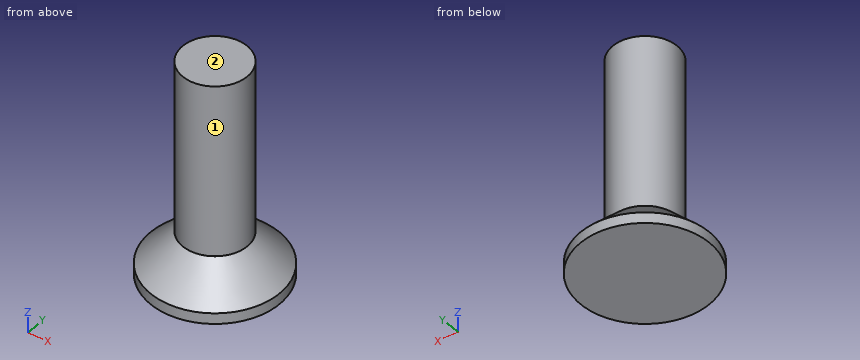
Autodesk Inventor part; units mm, degrees
ref_plane "YZ Plane" through (0, 0, 0) normal (1, 0, 0) x (0, 1, 0)
ref_plane "XZ Plane" through (0, 0, 0) normal (0, 1, 0) x (-1, 0, 0)
ref_plane "XY Plane" through (0, 0, 0) normal (0, 0, 1) x (1, 0, 0)
sketch "スケッチ1" plane through (0, 0, 0) normal (0, 0, 1) x (1, 0, 0)
  circle A0 centre (0, 0) radius 1.5
  dimension "d0" = 3
extrude "押し出し1" add sketch "スケッチ1" along normal blind 10
sketch "スケッチ2" plane through (0, 0, 0) normal (0, 0, -1) x (-1, 0, 0)
  circle A0 centre (0, 0) radius 3
  dimension "d3" = 6
extrude "押し出し2" add sketch "スケッチ2" against normal blind 2
thread "ねじ1"
chamfer "面取り1" distance 1.5 angle 45 1 edges at (3, 0, 2)
properties part number "ネジ皿m3,10" material "鋼、高強度、低合金"
Work out the finished part from the listing and answer in its coordinate system (mm). Face numbers are marked on the shaded views. A direction names the side the tool comes from. Give positions to 0.01 mm unless a question says otherwise; leave off trailing zeros. Order: outer loops, then holes, each group sorted by start corner. A loop starts at its lowest first (then second) coordinate and runs counter-clockwise, first axis right, second up. Notation, with made-up numbers: (41, 9.5) - (61, 9.5) arc R23 cw to (61, 24.5) - close; hole circle Ø6 at (13.25, 33.5). An arc over 180 degrees is marked (long way). Answer as CSV lines item,"result". Start each with the question number.
Q1. Given pin 1 Ø2 at (y, z) = (1.5, 3) entering from +X; pin 2 Ø1 at (x, z) = (0.5, 3) entering from -Y; pin 3 Ø1.5 at (x, y) = (2, -2) entering from +Z; pin 4 Ø3 at (x, y) = (0, -1.5) entering from -Z, each flat-ended and moving along its own axis, determine where each tip first touches the part or whether it passes through.
Q2. Find the intervals of material crossed by L1, parallel to Z at x = -2.15, y = -0.8; L2, parallel to Z at x = -0.85, y = -2.65; L3, parallel to Y at x = -1.15, z = 2.5, in increasing order. Write a range as [from, to].
Q3. For the marked faces 1 and 2, determine the directions among +Z, -Z, +X, -X, +Y, -Y from which every point of the face is accessible in a straight line to the end or side of a thin tool.
Q4. The part is cut by section C-C (z = 3.75). Write down the section's boundary in (x, y), then the cut area to 3 significant figures.
Check result:
1,pin 1,"stops at x = 1.41"
1,pin 2,"stops at y = -1.5"
1,pin 3,"stops at z = 1.42"
1,pin 4,"stops at z = 0"
2,L1,"z = [0, 1.21]"
2,L2,"z = [0, 0.72]"
2,L3,"y = [-0.96, 0.96]"
3,face 1,"+Z"
3,face 2,"+Z, +X, -X, +Y, -Y"
4,outline,"circle Ø3 at (0, 0)"
4,area,"7.07 mm²"
